Read the model definition and answer for the solid it produces. Units are mm, in the model's axes. Face numbers are marked on the shaded views. A direction names the side the tool comes from. Round coordinates to 2 decimals unless told otherwise and drop trailing zeros. Order: outer loops, then holes, each group sorted by start corner. A loop starts at its lowest first (then second) coordinate and runs counter-clockwise, first axis right, second up.
from build123d import *

# Parameters (mm, degrees)
SKETCH1_W           = 15
SKETCH1_H           = 15
BOSS_EXTRUDE1_DEPTH = 12
CUT_EXTRUDE1_DEPTH  = 2
CUT_EXTRUDE2_DEPTH  = 1.2
CUT_EXTRUDE3_DEPTH  = 8
SKETCH5_W           = 5.2
SKETCH5_H           = 12
BOSS_EXTRUDE2_DEPTH = 1
FILLET2_R           = 1
FILLET3_R           = 3
FILLET4_R           = 3


with BuildPart() as part:
    # Sketch1 → Boss-Extrude1 (new body)
    with BuildSketch(Plane(origin=(0, 0, 0), x_dir=(1, 0, 0), z_dir=(0, 1, 0))):
        Rectangle(SKETCH1_W, SKETCH1_H)
    extrude(amount=BOSS_EXTRUDE1_DEPTH)

    # Sketch2 → Cut-Extrude1 (cut)
    with BuildSketch(Plane(origin=(7.5, 0, 0), x_dir=(0, 0, -1), z_dir=(1, 0, 0))):
        Polygon((2.3, 10.4), (2.3, 9.6), (-2.3, 9.6), (-2.3, 10.4), (-2.3, 12), (2.3, 12), align=None)
    extrude(amount=-CUT_EXTRUDE1_DEPTH, mode=Mode.SUBTRACT)

    # Sketch3 → Cut-Extrude2 (cut)
    with BuildSketch(Plane(origin=(5.5, 0, 0), x_dir=(0, 0, -1), z_dir=(1, 0, 0))):
        with BuildLine():
            Line((-2.65, 11.29614814), (-2.65, 8.70385186))
            ThreePointArc((-2.65, 8.70385186), (0.665206735, 7.125978427), (2.95, 10))
            Line((2.95, 10), (2.95, 12))
            Line((2.95, 12), (-2.65, 12))
            Line((-2.65, 12), (-2.65, 11.29614814))
        make_face()
    extrude(amount=-CUT_EXTRUDE2_DEPTH, mode=Mode.SUBTRACT)

    # Sketch4 → Cut-Extrude3 (cut)
    with BuildSketch(Plane(origin=(4.3, 0, 0), x_dir=(0, 0, -1), z_dir=(1, 0, 0))):
        with BuildLine():
            Line((-2.55, 10), (-2.55, 12))
            Line((-2.55, 12), (2.55, 12))
            Line((2.55, 12), (2.55, 10))
            ThreePointArc((2.55, 10), (0, 7.45), (-2.55, 10))
        make_face()
    extrude(amount=-CUT_EXTRUDE3_DEPTH, mode=Mode.SUBTRACT)

    # Sketch5 → Boss-Extrude2 (add)
    with BuildSketch(Plane(origin=(7.5, 0, 0), x_dir=(0, 0, -1), z_dir=(1, 0, 0))):
        with Locations((4.9, 6)):
            Rectangle(SKETCH5_W, SKETCH5_H)
        with Locations((-4.9, 6)):
            Rectangle(SKETCH5_W, SKETCH5_H)
    extrude(amount=BOSS_EXTRUDE2_DEPTH)

    # Fillet2
    fillet2_edges = [part.edges().sort_by_distance(p)[0] for p in [
        (7.5, 9.6, 0),
    ]]
    fillet(fillet2_edges, radius=FILLET2_R)

    # Fillet3
    fillet3_edges = [part.edges().sort_by_distance(p)[0] for p in [
        (0.5, 12, -7.5),
        (-7.5, 12, 0),
        (8.5, 6, 7.5),
        (0.5, 12, 7.5),
        (-7.5, 6, -7.5),
        (8.5, 6, -7.5),
        (-7.5, 6, 7.5),
    ]]
    fillet(fillet3_edges, radius=FILLET3_R)

    # Fillet4
    # the kernel refuses this fillet: 3 mm, written as the material it takes off along each edge
    with BuildSketch(Plane(origin=(5.5, 9, 4.5), x_dir=(1, 0, 0), z_dir=(0, 1, 0))) as fillet4_piece_1_section:
        Polygon((0, 0), (FILLET4_R, 0), (FILLET4_R, -FILLET4_R), (0, -FILLET4_R), align=None)
    fillet4_piece_1 = extrude(amount=FILLET4_R, mode=Mode.PRIVATE)
    fillet4_piece_1 = fillet4_piece_1 - Plane(origin=(5.5, 9, 4.5), x_dir=(-0.7071067811865477, 0, -0.7071067811865475), z_dir=(0, 1, 0)) * Sphere(FILLET4_R, mode=Mode.PRIVATE)
    add(fillet4_piece_1, mode=Mode.SUBTRACT)
    with BuildSketch(Plane(origin=(5.5, 9, -4.5), x_dir=(1, 0, 0), z_dir=(0, 1, 0))) as fillet4_piece_2_section:
        Polygon((0, 0), (FILLET4_R, 0), (FILLET4_R, FILLET4_R), (0, FILLET4_R), align=None)
    fillet4_piece_2 = extrude(amount=FILLET4_R, mode=Mode.PRIVATE)
    fillet4_piece_2 = fillet4_piece_2 - Plane(origin=(5.5, 9, -4.5), x_dir=(-0.7071067811865475, 0, 0.7071067811865476), z_dir=(0, 1, 0)) * Sphere(FILLET4_R, mode=Mode.PRIVATE)
    add(fillet4_piece_2, mode=Mode.SUBTRACT)
    with BuildSketch(Plane(origin=(8.5, 12, -5.2), x_dir=(-1, 0, 0), z_dir=(0, 0, 1)), Plane(origin=(8.5, 12, -4.5), x_dir=(-1, 0, 0), z_dir=(0, 0, 1))) as fillet4_piece_3:
        with BuildLine():
            CenterArc((FILLET4_R, FILLET4_R), FILLET4_R, 180, 90)
            Line((0, FILLET4_R), (0, 0))
            Line((0, 0), (FILLET4_R, 0))
        make_face()
    extrude(amount=9.7, mode=Mode.SUBTRACT)


solid = part.part
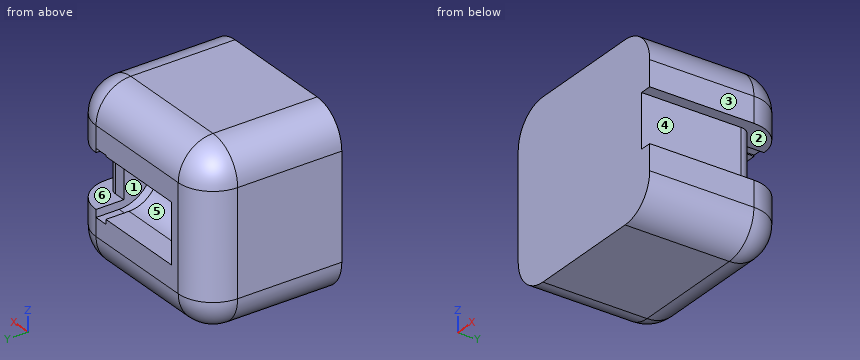
Q1. A cutting plane is placed at C-C, the plane z = 0. Give the vertices of the cut face in (x, y), plus the area to 3 significant figures.
Outcome:
outline: (-7.5, 0) - (7.5, 0) - (7.5, 8.6) arc R1 ccw to (6.5, 9.6) - (5.5, 9.6) - (5.5, 7.05) - (4.3, 7.05) - (4.3, 7.45) - (-3.7, 7.45) - (-3.7, 12) - (-4.5, 12) arc R3 ccw to (-7.5, 9) - close
area: 131 mm2
Q2. Flat-ended cylindrical pins translate along their axes: pin 1 (0.9 mm diameter, centred on x = 7.5, y = 7, fed in from -Z); pin 2 (1 mm diameter, centred on x = 5, y = 10, fed in from -Z); pin 3 (1.3 mm diameter, centred on x = 4.5, y = 11, fed in from +Z). Find the tip coordinate at first contact, or state that the pin passes through.
Outcome:
pin 1: stops at z = -7.07
pin 2: stops at z = -7.46
pin 3: stops at z = 7.18
Q3. A cutting plane is placed at D-D, the plane y = 9.25. Give the vertices of the cut face in (x, z).
Outcome:
outline: (-7.49, -4.5) arc R2.99 ccw to (-4.5, -7.49) - (5.5, -7.49) arc R2.99 ccw to (8.49, -4.5) - (8.49, -2.3) - (7.26, -2.3) - (7.26, 2.3) - (8.49, 2.3) - (8.49, 4.5) arc R2.99 ccw to (5.5, 7.49) - (-4.5, 7.49) arc R2.99 ccw to (-7.49, 4.5) - close; hole (-3.7, -2.44) - (4.3, -2.44) - (4.3, -2.85) - (5.5, -2.85) - (5.5, 2.65) - (4.3, 2.65) - (4.3, 2.44) - (-3.7, 2.44) - close
Q4. A cutting plane is placed at A-A, the plane x = -2.25. Give the vertices of the cut face in (y, z).
Outcome:
outline: (0, -7.5) - (9, -7.5) arc R3 ccw to (12, -4.5) - (12, -2.55) - (10, -2.55) arc R2.55 cw to (10, 2.55) - (12, 2.55) - (12, 4.5) arc R3 ccw to (9, 7.5) - (0, 7.5) - close
Q5. A cutting plane is placed at B-B, the plane y = 1.75. Give the vertices of the cut face in (x, z), plus the area to 3 significant figures.
Outcome:
outline: (-7.5, -4.5) arc R3 ccw to (-4.5, -7.5) - (5.5, -7.5) arc R3 ccw to (8.5, -4.5) - (8.5, -2.3) - (7.5, -2.3) - (7.5, 2.3) - (8.5, 2.3) - (8.5, 4.5) arc R3 ccw to (5.5, 7.5) - (-4.5, 7.5) arc R3 ccw to (-7.5, 4.5) - close
area: 228 mm2
Q6. For the marked faces 4, 5 and 6, determine the directions among +Z, -Z, +X, -X, +Y, -Y from which every point of the face is accessible in a straight line to the end or side of a thin tool.
Outcome:
face 4: +X, +Y, -Y
face 5: +Y
face 6: +X, +Y
Q7. For a pull along X with two mould halves and no side action, classify the marked faces 1, 2 and 3 as released by +X, released by -X, zero draft, split by the parting line, or undercut.
Outcome:
face 1: undercut
face 2: zero draft
face 3: released by +X
Q8. Straight lines are drawn through the part: probe 1 along X at (y, z) = (8.25, -1); probe 2 along X at (y, z) = (10, -2.5); probe 3 along X at (y, z) = (7.5, -2). For each, find the intervals that lie inside material, in ascending order.
Outcome:
probe 1: x = -7.5 to -3.7, 5.5 to 7.5
probe 2: x = -7.33 to -3.7, 5.5 to 8.33
probe 3: x = -7.5 to 7.5
